CAD build for the part. Positions are in the model's coordinates, mm. Give positions to 0.01 mm unless a question says otherwise; leave off trailing zeros. Order: outer loops, then holes, each group sorted by start corner. A loop starts at its lowest first (then second) coordinate and runs counter-clockwise, first axis right, second up. Notation, with made-up numbers: (61, -40) -> (108, -40) arc R25 ccw to (108, -21) -> close; hole circle Ø2 at (29, 8.25). An arc over 180 degrees is marked (long way). Use one line per item in the form item = value. Start each with the question number.
1) Mould opens along Z. For faces 1 (the face through (152, 0, -17)), 2 (the face through (22.368, 1.479, -23.849)), 3 (the face through (0.004, 1.479, -17.115)) say: pulls with the +Z half, pulls with the -Z half, needs draft (parallel to the pull), parting line crosses it, or undercut.
2) Probe line 1 (Z direction, x = 247.5, y = 0.65); line 2 (X direction, y = 2.8, z = -5.5); line 3 (X direction, y = 1.75, z = -29). List the from-to ranges inside material, lowest first.
3) Cut at A-A, the plane y = 0.55. State how many separate pieces and enclosed holes the cut face has, and give its area (3 significant figures).
4) Cut at B-B, the plane z = -23. Give the cut face in (x, y).
5) Drop flat-ended pins along their axis: P1, Ø1, axis at y = 2, z = -21.5, coming from the -X side; P2, Ø2.5, axis at x = 30.8, z = -7, coming from the +Y side. Give the stop position or say it passes through.
Autodesk Inventor part; units mm, degrees
ref_plane "YZ Plane" through (0, 0, 0) normal (1, 0, 0) x (0, 1, 0)
ref_plane "XZ Plane" through (0, 0, 0) normal (0, 1, 0) x (-1, 0, 0)
ref_plane "XY Plane" through (0, 0, 0) normal (0, 0, 1) x (1, 0, 0)
sketch "スケッチ1" plane through (0, 0, 0) normal (0, 1, 0) x (-1, 0, 0)
  line L0 (0, 0) -> (-300, 0)
  line L1 (-300, 0) -> (-300, -35)
  line L2 (-300, -35) -> (0, -35)
  line L3 (0, -35) -> (0, 0)
  arc A0 (-17.5, -35) -> (-17.5, 0) centre (-17.5, -17.5) ccw
  point P0 (-17.5, -17.5)
  dimension "d0" = 300
  dimension "d1" = 35
  dimension "d2" = 17.5
  dimension "d3" = 17.5
  dimension "d43" = 17.5
extrude "押し出し1" add sketch "スケッチ1" along normal blind 3 contours A0 L2 L1 L0
sketch "スケッチ2" plane through (0, 3, 0) normal (0, 1, 0) x (1, 0, 0)
  arc A0 (17.5, 35) -> (17.5, 0) centre (17.5, 17.5) ccw
  line L0 (300, 35) -> (17.5, 35)
  point P0 (0, 0)
  point P1 (0, 17.5)
hole "穴1" at (17.5, 3, -17.5) direction (0, -1, 0) diameter 16 end through all
sketch "スケッチ3" plane through (0, 3, 0) normal (0, 1, 0) x (1, 0, 0)
  line L0 (300, 0) -> (300, 35)
  arc A0 (17.5, 35) -> (17.5, 0) centre (17.5, 17.5) ccw construction
  line L1 (17.5, 17.5) -> (300, 17.5) construction
  line L2 (300, 0) -> (300, 35) construction
  point P0 (0, 0)
  point P1 (57.5, 17.5)
  point P2 (67.5, 17.5)
  point P3 (77.5, 17.5)
  point P4 (87.5, 17.5)
  point P5 (97.5, 17.5)
  point P6 (107.5, 17.5)
  point P7 (117.5, 17.5)
  point P8 (127.5, 17.5)
  point P9 (137.5, 17.5)
  point P10 (147.5, 17.5)
  point P11 (157.5, 17.5)
  point P12 (167.5, 17.5)
  point P13 (177.5, 17.5)
  point P14 (187.5, 17.5)
  point P15 (197.5, 17.5)
  point P16 (207.5, 17.5)
  point P17 (217.5, 17.5)
  point P18 (227.5, 17.5)
  point P19 (237.5, 17.5)
  point P20 (247.5, 17.5)
  point P21 (257.5, 17.5)
  point P22 (267.5, 17.5)
  point P23 (277.5, 17.5)
  point P24 (287.5, 17.5)
  dimension "d108" = 40
  dimension "d111" = 10
sketch "スケッチ8" plane through (0, 3, 0) normal (0, 1, 0) x (1, 0, 0)
  arc A0 (17.5, 35) -> (17.5, 0) centre (17.5, 17.5) ccw
  line L0 (0, 17.5) -> (37.6182, 17.5)
  line L1 (17.5, 0) -> (300, 0)
  circle A1 centre (15, 20) radius 8
  point P0 (0, 0)
  point P1 (30.8, 7)
  point P2 (30.8, 28)
  dimension "d84" = 17.5
  dimension "d85" = 10.5
  dimension "d86" = 10.5
  dimension "d88" = 15.8
  dimension "d89" = 15.8
hole "穴6" at (30.8, 3, -7) at (30.8, 3, -28) direction (0, -1, 0) diameter 3.3 end through all
hole "穴7" at (57.5, 3, -17.5) at (67.5, 3, -17.5) at (77.5, 3, -17.5) at (87.5, 3, -17.5) at (97.5, 3, -17.5) at (107.5, 3, -17.5) at (117.5, 3, -17.5) at (127.5, 3, -17.5) at (137.5, 3, -17.5) at (147.5, 3, -17.5) at (157.5, 3, -17.5) at (167.5, 3, -17.5) at (177.5, 3, -17.5) at (187.5, 3, -17.5) at (197.5, 3, -17.5) at (207.5, 3, -17.5) at (217.5, 3, -17.5) at (227.5, 3, -17.5) at (237.5, 3, -17.5) at (247.5, 3, -17.5) at (257.5, 3, -17.5) at (267.5, 3, -17.5) at (277.5, 3, -17.5) at (287.5, 3, -17.5) direction (0, -1, 0) diameter 3.2 end through all
properties part number "shoulder1_plate_top" material "アルミニウム 5052"
Result:
q1.face_1 = needs draft
q1.face_2 = undercut
q1.face_3 = parting line crosses it
q2.line_1 = -35 to -19.1, -15.9 to 0
q2.line_2 = 4.76 to 30.11, 31.49 to 300
q2.line_3 = 4.31 to 29.49, 32.11 to 300
q3.separate_pieces = 1
q3.enclosed_holes = 27
q3.area = 9,960 mm²
q4.outline = (0.89, 0) -> (11.69, 0) -> (11.69, 3) -> (0.89, 3) -> close; (23.31, 0) -> (300, 0) -> (300, 3) -> (23.31, 3) -> close
q5.P1 = 0.35
q5.P2 = through
